Source: CAD feature listing. Evaluate the final solid. Frame: model axes, mm. A direction names the side the tool comes from. Give positions to 0.01 mm unless a question says otherwise; leave off trailing zeros. Loops run counter-clockwise (first coordinate to the right, second up) from the corner with the lowest first, then second, coordinate; pieces in that order, holes last. Notation, with made-up numbers: (78, -12.5) - (91, -12.5) arc R24 cw to (91, 17.5) - close; hole circle Ø11 at (-15, 56). An arc over 180 degrees is marked (long way). Write each question's results on one line, items separated by ' | '. Start each with the question number.
(1) Cut plane B-B on x = -2. Return the cut outline in (y, z).
(2) Cut plane D-D on y = -4.75. Return the cut outline in (x, z).
(3) Cut plane C-C on y = -13.25. Return the cut outline in (x, z).
(4) Cut plane A-A on z = 0.7. Return the cut outline in (x, y), then the cut area to 3 significant figures.
(5) Reachability of faces 4 (the flat face through (0, -11, 1)), 5 (the flat face through (2.7, -12.3, 0.5)) from +Z, -Z, +X, -X, +Y, -Y: full face, straight path, thin tool, end or side. Return the list, or none.
(6) Pull-direction query (Y, two-part tool) for faces 1 (the flat face through (0, -11, 0)), 2 (the flat face through (2.266, -11.32, 0.493)), 3 (the flat face through (-9.4, -9.4, 0.5)); classes: pulls with the +Y half, pulls with the -Y half, needs draft (parallel to the pull), parting line crosses it, or undercut.
(7) Material intervals for line 1 along X through (y, z) = (-11, 0.25); line 2 along X through (y, z) = (-11.25, 0.2); line 3 along Y through (x, z) = (4, 0.1), sorted ascending. Write a range as [from, to].
from build123d import *

# Parameters (mm, degrees)
BOX092_W                  = 7.5
BOX092_H                  = 1
BOX092_DEPTH              = 2
BOX090_W                  = 7.5
BOX090_H                  = 1
BOX090_DEPTH              = 2
FUSION018_PLACEMENT_ANGLE = 45
EXTRUDE001_DEPTH          = 1


with BuildPart() as cube092:
    # Box092 → Box092 (new body)
    with BuildSketch(Plane.XY):
        with Locations((3.75, 0.5)):
            Rectangle(BOX092_W, BOX092_H)
    extrude(amount=BOX092_DEPTH)


with BuildPart() as obj1:
    # Box090 → Box090 (new body)
    with BuildSketch(Plane(origin=(1, 0, 0), x_dir=(0, 1, 0), z_dir=(0, 0, 1))):
        with Locations((3.75, 0.5)):
            Rectangle(BOX090_W, BOX090_H)
    extrude(amount=BOX090_DEPTH)

    # Fusion018: union Cube092
    add(cube092.part)


with BuildPart() as obj1_1:
    # Fusion018 placement: moved
    add(obj1.part.moved(Location((0, -15, 0))).rotate(Axis((0, -15, 0), (0, 0, 1)), FUSION018_PLACEMENT_ANGLE))


with BuildPart() as cut010:
    # Sketch012 → Extrude001 (new body)
    with BuildSketch(Plane.XY):
        Polygon((0, 0), (18.5, -18.5), (-18.5, -18.5), align=None)
    extrude(amount=EXTRUDE001_DEPTH)

    # Cut010: cut obj1
    add(obj1_1.part, mode=Mode.SUBTRACT)


solid = cut010.part
Ans:
1) outline: (-18.5, 0) - (-13, 0) - (-13, 1) - (-18.5, 1) - close; (-11.59, 0) - (-2, 0) - (-2, 1) - (-11.59, 1) - close
2) outline: (-4.75, 0) - (4.75, 0) - (4.75, 1) - (-4.75, 1) - close
3) outline: (-13.25, 0) - (-1.75, 0) - (-1.75, 1) - (-13.25, 1) - close; (-0.34, 0) - (0.34, 0) - (0.34, 1) - (-0.34, 1) - close; (1.75, 0) - (13.25, 0) - (13.25, 1) - (1.75, 1) - close
4) outline: (-18.5, -18.5) - (18.5, -18.5) - (0, 0) - close; hole (-5.3, -9.7) - (0, -15) - (5.3, -9.7) - (4.6, -8.99) - (0, -13.59) - (-4.6, -8.99) - close | area: 328 mm^2
5) face 4: +Z, +X, -X, +Y, -Y | face 5: +Z, -Z
6) face 1: needs draft | face 2: undercut | face 3: pulls with the +Y half
7) line 1: [-11, -4], [-2.59, 2.59], [4, 11] | line 2: [-11.25, -3.75], [-2.34, 2.34], [3.75, 11.25] | line 3: [-18.5, -11], [-9.59, -4]
